Part model, mm, in its own coordinate system. Face numbers are marked on the shaded views. Round coordinates to 2 decimals unless told otherwise and drop trailing zeros. Loops run counter-clockwise (first coordinate to the right, second up) from the corner with the lowest first, then second, coordinate; pieces in that order, holes last.
(1) Probe probe 1 along Y at (x, z) = (-9, -0.75); probe 2 along Y at (x, z) = (5, 6). List the from-to ranges inside material, lowest first.
(2) Mould opens along Y. For the marked faces 1, 2, 3 and 4 say: +Y half, -Y half, draft (parallel to the pull), parting line (faces both ways), or undercut.
(3) Cut at D-D on y = 2.85. List the corners of the cut face in (x, z).
(4) Cut at C-C on y = 1.4. List the corners of the cut face in (x, z), then the cut area to 3 significant figures.
Autodesk Inventor part; units mm, degrees
ref_plane "YZ Plane" through (0, 0, 0) normal (1, 0, 0) x (0, 1, 0)
ref_plane "XZ Plane" through (0, 0, 0) normal (0, 1, 0) x (-1, 0, 0)
ref_plane "XY Plane" through (0, 0, 0) normal (0, 0, 1) x (1, 0, 0)
sketch "Sketch1" plane through (0, 0, 0) normal (0, 1, 0) x (-1, 0, 0)
  circle A0 centre (0, 0) radius 10.16
  dimension "d0" = 20.32
extrude "Extrusion1" add sketch "Sketch1" along normal blind 2.54
chamfer "Chamfer1" distance 6.35 distance2 2.54 1 edges at (10.16, 2.54, 0) measured on face at (-6.5114, 2.54, 0.3794)
sketch "Sketch2" plane through (0, 2.54, 0) normal (0, 1, 0) x (1, 0, 0)
  circle A0 centre (0, 0) radius 10.16
extrude "Extrusion2" add sketch "Sketch2" along normal blind 2.54
chamfer "Chamfer2" distance 6.35 distance2 2.54 1 edges at (-10.16, 2.54, 0) measured on face at (7.9081, 2.54, 1.1144)
sketch "Sketch3" plane through (0, 0, 0) normal (0, -1, 0) x (1, 0, 0)
  circle A0 centre (0, 0) radius 3.81
  circle A1 centre (0, 0) radius 2.54
  dimension "d11" = 5.08
extrude "Extrusion3" cut sketch "Sketch3" against normal blind 5.08 contours A1
properties part number "Pulley"
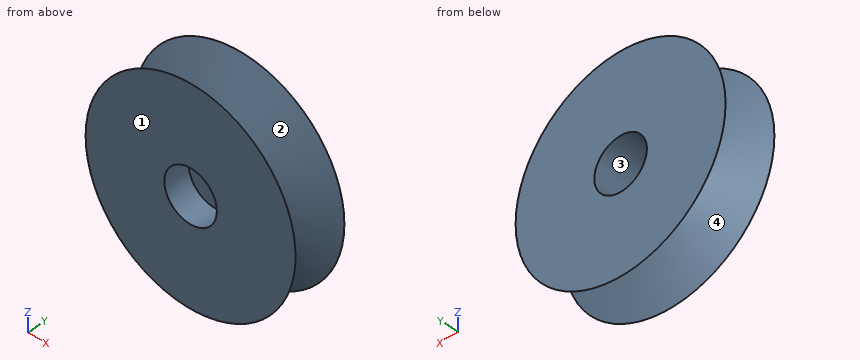
Final values:
1. probe 1: y = 0 to 0.45, 4.63 to 5.08
1. probe 2: y = 0 to 0.94, 4.14 to 5.08
2. face 1: -Y half
2. face 2: undercut
2. face 3: draft
2. face 4: undercut
3. outline: circle Ø9.17 at (0, 0); hole circle Ø5.08 at (0, 0)
4. outline: circle Ø13.32 at (0, 0); hole circle Ø5.08 at (0, 0)
4. area: 119 mm2
